from build123d import *

# Parameters (mm, degrees)
F0_R     = 70
F1_DEPTH = 5
F2_R     = 5.25
F3_DEPTH = 25
F5_DEPTH = 25
F6_W     = 10
F6_H     = 5
F7_DEPTH = 10
F9_DEPTH = 75.4


with BuildPart() as f1:
    # F0 (on Top) → F1 (new body)
    with BuildSketch(Plane.XY):
        Circle(F0_R)
    extrude(amount=F1_DEPTH)

    # F2 (on face) → F3 (cut)
    with BuildSketch(Plane.XY.offset(5)):
        with Locations((-45, 0)):
            Circle(F2_R)
        with BuildLine():
            ThreePointArc((33.1841421179, 46.8794410023), (25.3091421179, 51.4260743721), (25.3091421179, 42.3328076324))
            ThreePointArc((25.3091421179, 42.3328076324), (30.5591421179, 42.3328076324), (33.1841421179, 46.8794410023))
        make_face()
        with BuildLine():
            ThreePointArc((32.75, -47.6313972081), (30.125, -43.0847638383), (24.875, -43.0847638383))
            ThreePointArc((24.875, -43.0847638383), (24.875, -52.178030578), (32.75, -47.6313972081))
        make_face()
    extrude(amount=-F3_DEPTH, mode=Mode.SUBTRACT)

    # F4 (on face) → F5 (cut)
    with BuildSketch(Plane.XY.offset(5)):
        with BuildLine():
            Line((65.3834841531, 25), (0, 25))
            Line((0, 25), (0, -25))
            Line((0, -25), (65.3834841531, -25))
            ThreePointArc((65.3834841531, -25), (68.8361964766, -12.7113356749), (70, 0))
            ThreePointArc((70, 0), (68.8361964766, 12.7113356749), (65.3834841531, 25))
        make_face()
    extrude(amount=-F5_DEPTH, mode=Mode.SUBTRACT)

    # F6 (on face) → F7 (join)
    with BuildSketch(Plane(origin=(0, 0, 0), x_dir=(1, 0, 0), z_dir=(0, 0, -1))):
        with Locations((21, -27.5)):
            Rectangle(F6_W, F6_H)
        with Locations((21, 27.5)):
            Rectangle(F6_W, F6_H)
    extrude(amount=F7_DEPTH)

    # F8 (on face) → F9 (cut)
    with BuildSketch(Plane(origin=(0, 30, 0), x_dir=(-1, 0, 0), z_dir=(0, 1, 0))):
        with BuildLine():
            Line((-21, -5), (-22.767766953, -3.232233047))
            ThreePointArc((-22.767766953, -3.232233047), (-23.5, -5), (-22.767766953, -6.767766953))
            Line((-22.767766953, -6.767766953), (-21, -5))
        make_face()
        with BuildLine():
            Line((-19.232233047, -3.232233047), (-21, -5))
            Line((-21, -5), (-19.232233047, -6.767766953))
            ThreePointArc((-19.232233047, -6.767766953), (-18.6903011687, -5.9567085809), (-18.5, -5))
            ThreePointArc((-18.5, -5), (-18.6903011687, -4.0432914191), (-19.232233047, -3.232233047))
        make_face()
        with BuildLine():
            Line((-19.232233047, -6.767766953), (-21, -5))
            Line((-21, -5), (-22.767766953, -6.767766953))
            ThreePointArc((-22.767766953, -6.767766953), (-21, -7.5), (-19.232233047, -6.767766953))
        make_face()
        with BuildLine():
            ThreePointArc((-19.232233047, -3.232233047), (-21, -2.5), (-22.767766953, -3.232233047))
            Line((-22.767766953, -3.232233047), (-21, -5))
            Line((-21, -5), (-19.232233047, -3.232233047))
        make_face()
    extrude(amount=-F9_DEPTH, mode=Mode.SUBTRACT)


solid = f1.part
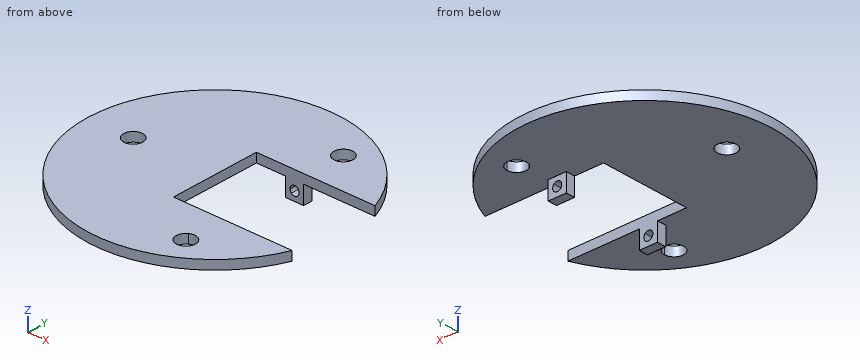
The model under review builds one solid part; all positions refer to its coordinate system, in mm. Round coordinates to 2 decimals unless told otherwise and drop trailing zeros. Write each loop counter-clockwise with the first axis right and the second up, starting at its lowest first coordinate (ties: lowest second). Pieces come first, ordered by that corner, then holes. Notation, with made-up numbers: (-12.5, 29) -> (21.5, 29) arc R25 cw to (21.5, 54) -> close; hole circle Ø8 at (67, 35.5). An arc over 180 degrees is marked (long way). Answer as a JSON object with one key per item and string values.
1. Clearance check with flat-ended pins moving along their axes: pin 1 (4 mm diameter, centred on y = -26.5, z = -3.5, fed in from +X); pin 2 (4 mm diameter, centred on y = 27, z = -6.5, fed in from -X); pin 3 (12 mm diameter, centred on x = 27.5, y = -47.63, fed in from +Z); pin 4 (8 mm diameter, centred on x = 26, z = -5.5, fed in from -Y). State where each tip first meets the part, or that it passes through.
Results found:
{"pin 1": "stops at x = 26", "pin 2": "stops at x = 16", "pin 3": "stops at z = 5", "pin 4": "stops at y = -30"}
2. We need section A-A on z = 3. State the section outline as (x, y) points (3 decimals), and give its area (3 significant figures).
Results found:
{"outline": "(0, -25) -> (0, 25) -> (65.383, 25) arc R70 ccw (long way) to (65.383, -25) -> close; hole circle Ø10.5 at (-45, 0); hole circle Ø10.5 at (27.5, -47.631); hole circle Ø10.5 at (27.934, 46.879)", "area": "11,700 mm^2"}
3. We need section D-D on x = -16.5. State the section outline as (y, z) points, and give its area (3 significant figures).
Results found:
{"outline": "(-68.03, 0) -> (68.03, 0) -> (68.03, 5) -> (-68.03, 5) -> close", "area": "680 mm^2"}
4. We need section C-C on x = -45. State the section outline as (y, z) points.
Results found:
{"outline": "(-53.62, 0) -> (-5.25, 0) -> (-5.25, 5) -> (-53.62, 5) -> close; (5.25, 0) -> (53.62, 0) -> (53.62, 5) -> (5.25, 5) -> close"}
5. To check wall thickness, follow line 1 along Y through (x, z) = (27.5, 2.75); line 2 along Z through (x, y) = (-5, -6); line 3 along X through (y, z) = (-4, 0.75). State the ranges of each line that lie inside material, in increasing order.
Results found:
{"line 1": "y = -64.37 to -52.88, -42.38 to -25, 25 to 41.65, 52.11 to 64.37", "line 2": "z = 0 to 5", "line 3": "x = -69.89 to -48.4, -41.6 to 0"}
6. We need section B-B on y = 0. State the section outline as (x, z) points.
Results found:
{"outline": "(-70, 0) -> (-50.25, 0) -> (-50.25, 5) -> (-70, 5) -> close; (-39.75, 0) -> (0, 0) -> (0, 5) -> (-39.75, 5) -> close"}
